```python
from build123d import *

# Parameters (mm, degrees)
F0_R     = 11
F0_R_2   = 5.5
F1_DEPTH = 2.5
F0_R_3   = 4.05
F2_DEPTH = 3.2
F3_DEPTH = 6.2
F4_R     = 2.49999
F5_R     = 0.5


# Not quite as in the source:
# - a fillet or chamfer is up to 0.001 mm smaller than in the source, because OpenCascade refuses the exact size


with BuildPart() as f1:
    # F0 (on Top) → F1 (new body)
    with BuildSketch(Plane.XY):
        Circle(F0_R)
        Circle(F0_R_2, mode=Mode.SUBTRACT)
    extrude(amount=F1_DEPTH)

    # F0 (on Top) → F2 (join)
    with BuildSketch(Plane.XY):
        Circle(F0_R_2)
        Circle(F0_R_3, mode=Mode.SUBTRACT)
    extrude(amount=F2_DEPTH)

    # F0 (on Top) → F3 (join)
    with BuildSketch(Plane.XY):
        Circle(F0_R_3)
    extrude(amount=F3_DEPTH)

    # F4 (radius 2.5 in the source; OpenCascade refuses exactly that, so slightly less here)
    f4_edges = [f1.edges().sort_by_distance(p)[0] for p in [
        (-11, 0, 0),
    ]]
    fillet(f4_edges, radius=F4_R)

    # F5
    f5_edges = [f1.edges().sort_by_distance(p)[0] for p in [
        (-4.05, 0, 6.2),
    ]]
    fillet(f5_edges, radius=F5_R)


solid = f1.part
```
Verification items for the finished model (mm, model axes). A direction names the side the tool comes from. Round coordinates to 2 decimals unless told otherwise and drop trailing zeros. Order: outer loops, then holes, each group sorted by start corner. A loop starts at its lowest first (then second) coordinate and runs counter-clockwise, first axis right, second up. Notation, with made-up numbers: (-35.5, -30.75) - (22.5, -30.75) arc R21 ccw to (22.5, 1.25) - close; hole circle Ø6 at (80.25, 58). An arc over 180 degrees is marked (long way). Use CSV: the item, a comma, the result in double quotes. Start each with the question number.
1) Access from +Z, -Z, +X, -X, +Y, -Y to the whole of each face (thin tool, end or side, straight path). Record for faces 3 (the cylindrical face through (-0.878, -3.954, 4.432)), 4 (the flat face through (0, 0, 6.2)).
2) Section check D-D, the plane z = 1.5. Record the cut outline in (x, y), plus the area to 3 significant figures.
3) Mould release check, pull along X, two halves, no side actions. Record for faces 1 (the cylindrical face through (-1.19, -5.37, 2.85)), 2 (the flat face through (-3, 5, 2.5)): +X half, -X half, draft (parallel to the pull), parting line (faces both ways), or undercut.
4) Thickness scan on L1, parallel to Z at x = 7.75, y = 1; L2, parallel to Y at x = -9, z = 1.5; L3, parallel to X at y = 6, z = 1.5. Record the ranges inside material, lowest first.
5) Go/stop test with flat-tipped pins: P1, Ø3, axis at x = -5.5, z = 1.5, coming from the +Y side; P2, Ø3, axis at x = 1, y = -6, coming from the +Z side. Record where each tip stops, or that it passes through.
6) Section check C-C, the plane z = 4.5. Record the cut outline in (x, y).
Answers:
1,face 3,"+Z"
1,face 4,"+Z, +X, -X, +Y, -Y"
2,outline,"circle Ø21.58 at (0, 0)"
2,area,"366 mm²"
3,face 1,"parting line"
3,face 2,"draft"
4,L1,"z = 0 to 2.5"
4,L2,"y = -5.95 to 5.95"
4,L3,"x = -8.97 to 8.97"
5,P1,"stops at y = 10.16"
5,P2,"stops at z = 3.2"
6,outline,"circle Ø8.1 at (0, 0)"
